Check sheet for the modelled part. Datum: model origin and axes. Units: mm. Face numbers are marked on the shaded views. A direction names the side the tool comes from. Coordinates: 2 decimals unless noted, no trailing zeros. Write each loop counter-clockwise with the first axis right and the second up, starting at its lowest first coordinate (ties: lowest second). Pieces come first, ordered by that corner, then holes. Notation, with made-up numbers: (37.25, 61.5) -> (54.25, 61.5) arc R21 ccw to (54.25, 67.5) -> close; hole circle Ø11 at (21.5, 67). An arc over 180 degrees is marked (long way). One line per item, written item: value. Start each with the question number.
1) Draft check along Y on the marked faces 1, 2, 3 and 4. Enter one of: +Y half, -Y half, draft (parallel to the pull), parting line (faces both ways), or undercut.
2) Scan lines: line 1 along X through (y, z) = (1.7, 6); line 2 along Z through (x, y) = (12, 29); line 3 along Z through (x, y) = (8.75, 14). Record each from-to range of solid material in increasing order. Write a range as [from, to].
3) Sectioned sample at B-B on z = -3.75. Enter the section's corners in (x, y), plus the area to 3 significant figures.
4) Sectioned sample at D-D on z = 6. Enter the section's corners in (x, y).
5) Set-up check for the marked faces 5, 6 and 7: record each of +Z, -Z, +X, -X, +Y, -Y from which the full face is reachable in a straight line by a thin tool's end or side.
6) Gauge pin test, flat ends, axial feed: P1, Ø19, axis at x = -13.5, y = 32.5, coming from the +Z side; P2, Ø4, axis at y = 26, z = -4.5, coming from the -X side; P3, Ø2, axis at x = 13.5, z = 1, coming from the +Y side; P4, Ø5, axis at x = 27.5, z = 6, coming from the -Y side. Record the tip position at first contact, or that the pin passes through.
7) Sectioned sample at A-A on x = -7. Enter the section's corners in (y, z), plus the area to 3 significant figures.
8) Sectioned sample at C-C on y = 20.5. Enter the section's corners in (x, z), plus the area to 3 significant figures.
```python
from build123d import *

# Parameters (mm, degrees)
SKETCH1_R                 = 1.5
BOSS_EXTRUDE1_DEPTH       = 3
SKETCH3_R                 = 14.5
BOSS_EXTRUDE2_DEPTH       = 14
M3X0_5_TAPPED_HOLE1_D     = 2.5
M3X0_5_TAPPED_HOLE1_DEPTH = 10.748924226
M3X0_5_TAPPED_HOLE1_TIP   = 0.751075774
FILLET2_R                 = 0.5


with BuildPart() as part:
    # Sketch1 → Boss-Extrude1 (new body)
    with BuildSketch(Plane(origin=(0, 0, 0), x_dir=(1, 0, 0), z_dir=(0, 1, 0))):
        with BuildLine():
            Line((-29.5, -11), (29.5, -11))
            ThreePointArc((29.5, -11), (31.621320344, -10.121320344), (32.5, -8))
            Line((32.5, -8), (32.5, 8))
            ThreePointArc((32.5, 8), (31.621320344, 10.121320344), (29.5, 11))
            Line((29.5, 11), (-29.5, 11))
            ThreePointArc((-29.5, 11), (-31.621320344, 10.121320344), (-32.5, 8))
            Line((-32.5, 8), (-32.5, -8))
            ThreePointArc((-32.5, -8), (-31.621320344, -10.121320344), (-29.5, -11))
        make_face()
        with Locations(Location((-27.5, -6, 0), (0, 0, 270))):
            Circle(SKETCH1_R, mode=Mode.SUBTRACT)
        with Locations(Location((27.5, -6, 0), (0, 0, 270))):
            Circle(SKETCH1_R, mode=Mode.SUBTRACT)
    extrude(amount=BOSS_EXTRUDE1_DEPTH)

    # Sketch3 → Boss-Extrude2 (add)
    with BuildSketch(Plane(origin=(0, 0, -11), x_dir=(-1, 0, 0), z_dir=(0, 0, -1))):
        with BuildLine():
            Line((24.5, 3), (24.5, 44.5))
            ThreePointArc((24.5, 44.5), (7, 62), (-10.5, 44.5))
            Line((-10.5, 44.5), (-10.5, 35))
            Line((-10.5, 35), (-15, 35))
            Line((-15, 35), (-15, 3))
            Line((-15, 3), (24.5, 3))
        make_face()
        with Locations((7, 44.5)):
            Circle(SKETCH3_R, mode=Mode.SUBTRACT)
    extrude(amount=-BOSS_EXTRUDE2_DEPTH)

    # M3x0.5 Tapped Hole1
    with Locations(Plane(origin=(15, 0, 0), x_dir=(0, 0, -1), z_dir=(1, 0, 0))):
        with Locations((0, 14), (8, 29)):
            Hole(M3X0_5_TAPPED_HOLE1_D / 2, depth=M3X0_5_TAPPED_HOLE1_DEPTH)
            with Locations((0, 0, -(M3X0_5_TAPPED_HOLE1_DEPTH + M3X0_5_TAPPED_HOLE1_TIP / 2))):  # 118° drill point
                Cone(0, M3X0_5_TAPPED_HOLE1_D / 2, M3X0_5_TAPPED_HOLE1_TIP, mode=Mode.SUBTRACT)

    # Fillet2
    fillet2_edges = [part.edges().sort_by_distance(p)[0] for p in [
        (-31.621320344, 3, -10.121320344),
        (-32.5, 3, 0),
        (-31.621320344, 3, 10.121320344),
        (0, 3, 11),
        (31.621320344, 3, 10.121320344),
        (32.5, 3, 0),
        (-27, 3, -11),
        (-24.5, 23.75, -11),
        (-24.5, 3, -4),
        (15, 19, 3),
        (15, 3, -4),
        (12.75, 35, 3),
        (15, 35, -4),
        (10.5, 39.75, 3),
        (10.5, 35, -4),
        (-7, 62, 3),
        (-24.5, 23.75, 3),
        (-4.75, 3, 3),
        (-7, 62, -11),
        (10.5, 39.75, -11),
        (12.75, 35, -11),
        (15, 19, -11),
        (31.621320344, 3, -10.121320344),
        (22.25, 3, -11),
    ]]
    fillet(fillet2_edges, radius=FILLET2_R)


solid = part.part
```
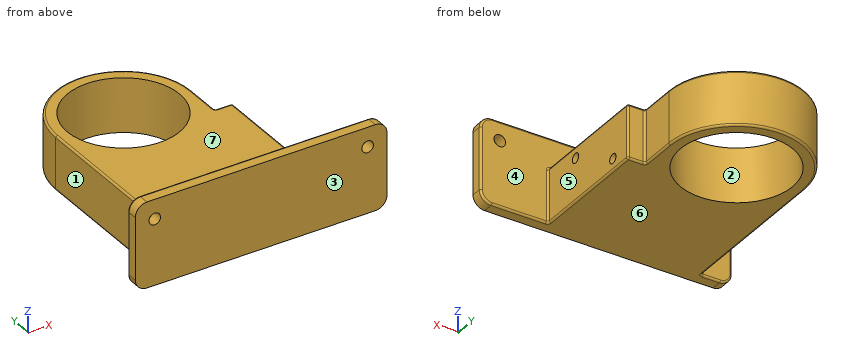
Answers:
1. face 1: draft
1. face 2: undercut
1. face 3: -Y half
1. face 4: +Y half
2. line 1: x = [-32.5, -29], [-26, 26], [29, 32.5]
2. line 2: z = [-11, -9.25], [-6.75, 3]
2. line 3: z = [-11, -1.25], [1.25, 3]
3. outline: (-32.5, 0) -> (32.5, 0) -> (32.5, 2.5) arc R0.5 ccw to (32, 3) -> (15.5, 3) arc R0.5 cw to (15, 3.5) -> (15, 34.5) arc R0.5 ccw to (14.5, 35) -> (11, 35) arc R0.5 cw to (10.5, 35.5) -> (10.5, 44.5) arc R17.5 ccw to (-24.5, 44.5) -> (-24.5, 3.5) arc R0.5 cw to (-25, 3) -> (-32, 3) arc R0.5 ccw to (-32.5, 2.5) -> close; hole circle Ø29 at (-7, 44.5)
3. area: 1,610 mm2
4. outline: (-32.5, 0) -> (-29, 0) -> (-29, 3) -> (-32, 3) arc R0.5 ccw to (-32.5, 2.5) -> close; (-26, 0) -> (26, 0) -> (26, 3) -> (-26, 3) -> close; (29, 0) -> (32.5, 0) -> (32.5, 2.5) arc R0.5 ccw to (32, 3) -> (29, 3) -> close
5. face 5: +Z, -Z, +X, +Y
5. face 6: -Z, +X, -X, +Y, -Y
5. face 7: +Z, +X, -X, +Y
6. P1: stops at z = 3
6. P2: stops at x = -24.5
6. P3: stops at y = 35
6. P4: stops at y = 0
7. outline: (0, -11) -> (30, -11) -> (30, 3) -> (3.5, 3) arc R0.5 cw to (3, 3.5) -> (3, 10.5) arc R0.5 ccw to (2.5, 11) -> (0, 11) -> close; (59, -11) -> (61.5, -11) arc R0.5 ccw to (62, -10.5) -> (62, 2.5) arc R0.5 ccw to (61.5, 3) -> (59, 3) -> close
7. area: 486 mm2
8. outline: (-24.5, -10.5) arc R0.5 ccw to (-24, -11) -> (14.5, -11) arc R0.5 ccw to (15, -10.5) -> (15, 2.5) arc R0.5 ccw to (14.5, 3) -> (-24, 3) arc R0.5 ccw to (-24.5, 2.5) -> close
8. area: 553 mm2
